Source: three-view drawing plus pictorial views. Frame: mm from the lowest corner of the part. A direction names the side the tool comes from. Coordinates: 2 decimals unless noted, no trailing zeros. Order: outer loops, then holes, each group sorted by start corner. A loop starts at its lowest first (then second) coordinate and runs counter-clockwise, first axis right, second up. Notation, with made-up numbers: (-9, 41) -> (28, 41) arc R6 cw to (28, 45) -> close; hole circle Ø6 at (16, 23.5). An arc over 180 degrees is marked (long way). One line per question, with ' | ' between items.
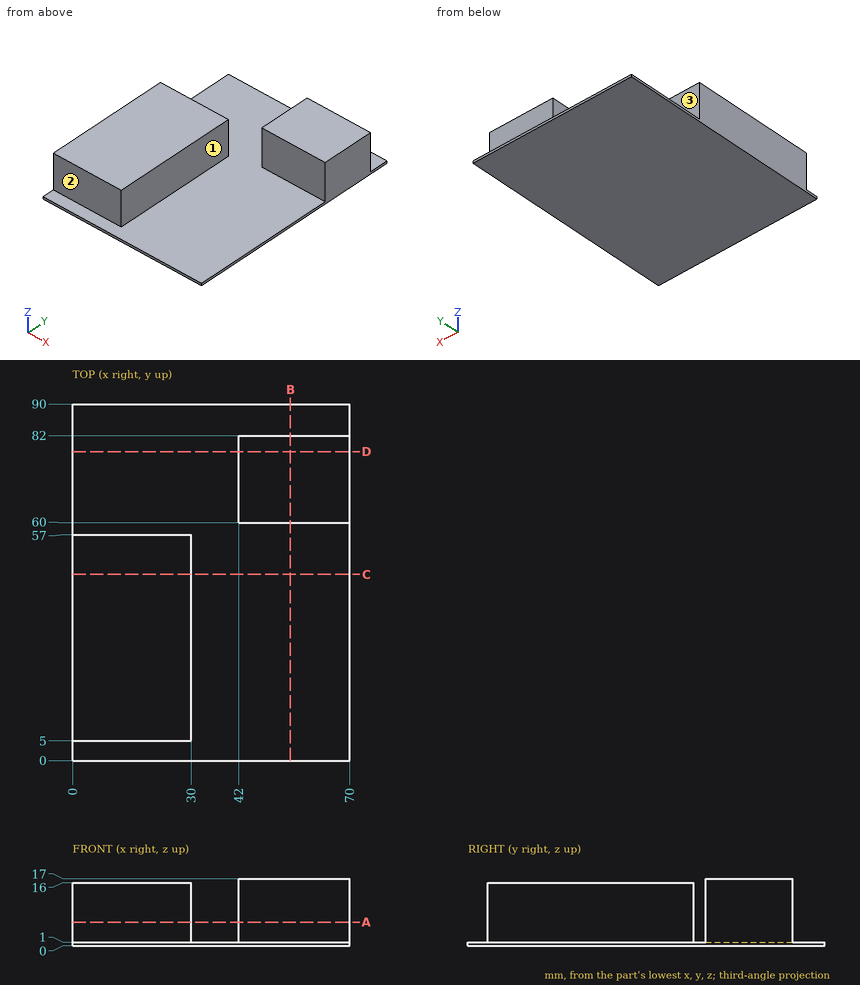
1. Pin query (flat end, axial travel): pin 1 Ø1.5 at (x, y) = (13, 17.5) entering from +Z; pin 2 Ø2 at (x, z) = (14, 8) entering from +Y; pin 3 Ø4.5 at (y, z) = (31, 11) entering from +X. Return the tip coordinate at first contact, or that it passes through.
Recorded:
pin 1: stops at z = 16 | pin 2: stops at y = 57 | pin 3: stops at x = 30
2. Access query for the marked faces 1, 2 and 3. Directions: +Z, -Z, +X, -X, +Y, -Y. A direction counts if a zero-diameter tool reaches every point of the face in a straight line with its end or side. Return the directions, or none.
Recorded:
face 1: +Z, +X, +Y, -Y | face 2: +Z, +X, -X, -Y | face 3: +Z, +X, -X, +Y
3. Cut plane C-C, the plane y = 47. Return loops of the section in (x, z).
Recorded:
outline: (0, 0) -> (70, 0) -> (70, 1) -> (30, 1) -> (30, 16) -> (0, 16) -> close
4. Cut plane A-A, the plane z = 6. Return loops of the section in (x, y).
Recorded:
outline: (0, 5) -> (30, 5) -> (30, 57) -> (0, 57) -> close; (42, 60) -> (70, 60) -> (70, 82) -> (42, 82) -> close
5. Ray query, line 1 (Z direction, x = 13, y = 10); line 2 (Y direction, x = 10, z = 13.5); line 3 (Z direction, x = 59, y = 84.5). Return the intervals inside material, ascending. Write a range as [from, to].
Recorded:
line 1: z = [0, 16] | line 2: y = [5, 57] | line 3: z = [0, 1]
6. Cut plane B-B, the plane x = 55. Return loops of the section in (y, z).
Recorded:
outline: (0, 0) -> (90, 0) -> (90, 1) -> (82, 1) -> (82, 17) -> (60, 17) -> (60, 1) -> (0, 1) -> close
7. Cut plane D-D, the plane y = 78. Return loops of the section in (x, z), and give its area (3 significant figures).
Recorded:
outline: (0, 0) -> (70, 0) -> (70, 17) -> (42, 17) -> (42, 1) -> (0, 1) -> close | area: 518 mm^2
